Input: part model. Units: mm. Frame: model coordinates. Face numbers are marked on the shaded views. Coordinates: 2 decimals unless noted, no trailing zeros. Write each loop counter-clockwise with the first axis right and the second up, starting at its lowest first coordinate (ties: lowest second). Pieces come first, ordered by that corner, then holes. Notation, with made-up numbers: M -13,-40 L -6,-40 A6 ccw -6,-36 Z; hole C 24,-25 d2. An arc over 180 degrees is marked long. Use one line per item in the form item = value.
from build123d import *

# Parameters (mm, degrees)
SKETCH_1_R      = 46
SKETCH_1_R_2    = 20
SKETCH_1_R_3    = 3.1
EXTRUDE_1_DEPTH = 4
EXTRUDE_START   = 4
SKETCH_1_8_R    = 46
SKETCH_1_8_R_2  = 3.1
SKETCH_1_8_R_3  = 20
SKETCH_1_8_R_4  = 2.6
EXTRUDE_3_DEPTH = 6


with BuildPart() as part:
    # 草图1 → 凸台-拉伸1 (new body)
    with BuildSketch(Plane(origin=(0, 0, 0), x_dir=(1, 0, 0), z_dir=(0, 1, 0))):
        with Locations(Location((0, 0, 0), (0, 0, 270))):
            Circle(SKETCH_1_R)
        with Locations(Location((0, 0, 0), (0, 0, 270))):
            Circle(SKETCH_1_R_2, mode=Mode.SUBTRACT)
        with Locations(Location((0, 41, 0), (0, 0, 270))):
            Circle(SKETCH_1_R_3, mode=Mode.SUBTRACT)
        with Locations(Location((41, 0, 0), (0, 0, 270))):
            Circle(SKETCH_1_R_3, mode=Mode.SUBTRACT)
        with Locations(Location((0, -41, 0), (0, 0, 270))):
            Circle(SKETCH_1_R_3, mode=Mode.SUBTRACT)
        with Locations(Location((-41, 0, 0), (0, 0, 270))):
            Circle(SKETCH_1_R_3, mode=Mode.SUBTRACT)
        Polygon((-19.45, 21.16173141), (-19.45, 25.83826859), (-23.5, 28.17653718), (-27.55, 25.83826859), (-27.55, 21.16173141), (-23.5, 18.82346282), align=None, mode=Mode.SUBTRACT)
        Polygon((21.16173141, 19.45), (25.83826859, 19.45), (28.17653718, 23.5), (25.83826859, 27.55), (21.16173141, 27.55), (18.82346282, 23.5), align=None, mode=Mode.SUBTRACT)
        Polygon((19.45, -21.16173141), (19.45, -25.83826859), (23.5, -28.17653718), (27.55, -25.83826859), (27.55, -21.16173141), (23.5, -18.82346282), align=None, mode=Mode.SUBTRACT)
        Polygon((-21.16173141, -19.45), (-25.83826859, -19.45), (-28.17653718, -23.5), (-25.83826859, -27.55), (-21.16173141, -27.55), (-18.82346282, -23.5), align=None, mode=Mode.SUBTRACT)
    extrude(amount=EXTRUDE_1_DEPTH)

    # 草图1<8> → 凸台-拉伸3 (add)
    # profile 1 of 5: a face of its own
    with BuildSketch(Plane(origin=(0, 0, 0), x_dir=(1, 0, 0), z_dir=(0, 1, 0)).offset(EXTRUDE_START)):
        with Locations(Location((0, 0, 0), (0, 0, 270))):
            Circle(SKETCH_1_8_R)
        with Locations(Location((-41, 0, 0), (0, 0, 270))):
            Circle(SKETCH_1_8_R_2, mode=Mode.SUBTRACT)
        with Locations(Location((0, -41, 0), (0, 0, 270))):
            Circle(SKETCH_1_8_R_2, mode=Mode.SUBTRACT)
        with Locations(Location((41, 0, 0), (0, 0, 270))):
            Circle(SKETCH_1_8_R_2, mode=Mode.SUBTRACT)
        with Locations(Location((0, 41, 0), (0, 0, 270))):
            Circle(SKETCH_1_8_R_2, mode=Mode.SUBTRACT)
        with Locations(Location((0, 0, 0), (0, 0, 270))):
            Circle(SKETCH_1_8_R_3, mode=Mode.SUBTRACT)
        Polygon((-23.5, 18.82346282), (-19.45, 21.16173141), (-19.45, 25.83826859), (-23.5, 28.17653718), (-27.55, 25.83826859), (-27.55, 21.16173141), align=None, mode=Mode.SUBTRACT)
        Polygon((18.82346282, 23.5), (21.16173141, 19.45), (25.83826859, 19.45), (28.17653718, 23.5), (25.83826859, 27.55), (21.16173141, 27.55), align=None, mode=Mode.SUBTRACT)
        Polygon((23.5, -18.82346282), (19.45, -21.16173141), (19.45, -25.83826859), (23.5, -28.17653718), (27.55, -25.83826859), (27.55, -21.16173141), align=None, mode=Mode.SUBTRACT)
        Polygon((-18.82346282, -23.5), (-21.16173141, -19.45), (-25.83826859, -19.45), (-28.17653718, -23.5), (-25.83826859, -27.55), (-21.16173141, -27.55), align=None, mode=Mode.SUBTRACT)
    # profile 2 of 5: a face of its own
    with BuildSketch(Plane(origin=(0, 0, 0), x_dir=(1, 0, 0), z_dir=(0, 1, 0)).offset(EXTRUDE_START)):
        Polygon((-21.16173141, -27.55), (-18.82346282, -23.5), (-21.16173141, -19.45), (-25.83826859, -19.45), (-28.17653718, -23.5), (-25.83826859, -27.55), align=None)
        with Locations(Location((-23.5, -23.5, 0), (0, 0, 270))):
            Circle(SKETCH_1_8_R_4, mode=Mode.SUBTRACT)
    # profile 3 of 5: a face of its own
    with BuildSketch(Plane(origin=(0, 0, 0), x_dir=(1, 0, 0), z_dir=(0, 1, 0)).offset(EXTRUDE_START)):
        Polygon((27.55, -21.16173141), (23.5, -18.82346282), (19.45, -21.16173141), (19.45, -25.83826859), (23.5, -28.17653718), (27.55, -25.83826859), align=None)
        with Locations(Location((23.5, -23.5, 0), (0, 0, 270))):
            Circle(SKETCH_1_8_R_4, mode=Mode.SUBTRACT)
    # profile 4 of 5: a face of its own
    with BuildSketch(Plane(origin=(0, 0, 0), x_dir=(1, 0, 0), z_dir=(0, 1, 0)).offset(EXTRUDE_START)):
        Polygon((21.16173141, 27.55), (18.82346282, 23.5), (21.16173141, 19.45), (25.83826859, 19.45), (28.17653718, 23.5), (25.83826859, 27.55), align=None)
        with Locations(Location((23.5, 23.5, 0), (0, 0, 270))):
            Circle(SKETCH_1_8_R_4, mode=Mode.SUBTRACT)
    # profile 5 of 5: a face of its own
    with BuildSketch(Plane(origin=(0, 0, 0), x_dir=(1, 0, 0), z_dir=(0, 1, 0)).offset(EXTRUDE_START)):
        Polygon((-27.55, 21.16173141), (-23.5, 18.82346282), (-19.45, 21.16173141), (-19.45, 25.83826859), (-23.5, 28.17653718), (-27.55, 25.83826859), align=None)
        with Locations(Location((-23.5, 23.5, 0), (0, 0, 270))):
            Circle(SKETCH_1_8_R_4, mode=Mode.SUBTRACT)
    extrude(amount=EXTRUDE_3_DEPTH)


solid = part.part
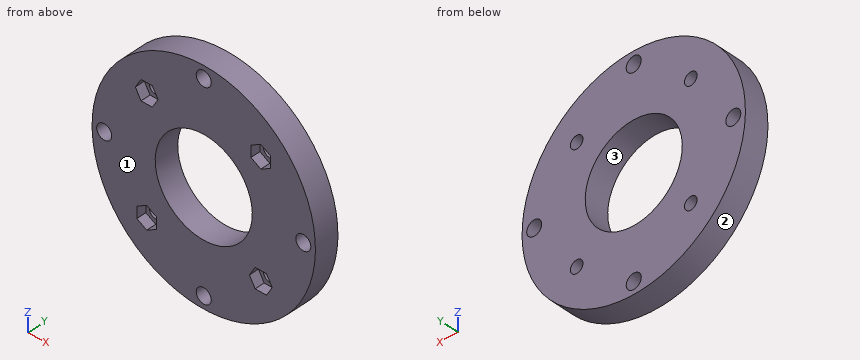
(1) Section query C-C on z = -41. Return the cut outline in (x, y), plus the area to 3 significant figures.
Computed:
outline = M -20.86,0 L -3.1,0 L -3.1,10 L -20.86,10 Z; M 3.1,0 L 20.86,0 L 20.86,10 L 3.1,10 Z
area = 355 mm^2
(2) Section query B-B on x = 0. Return the cut outline in (y, z).
Computed:
outline = M 0,-46 L 10,-46 L 10,-44.1 L 0,-44.1 Z; M 0,-37.9 L 10,-37.9 L 10,-20 L 0,-20 Z; M 0,20 L 10,20 L 10,37.9 L 0,37.9 Z; M 0,44.1 L 10,44.1 L 10,46 L 0,46 Z
(3) Section query A-A on y = 6.5. State how many separate pieces and enclosed holes the cut face has, plus the area to 3 significant figures.
Computed:
separate_pieces = 1
enclosed_holes = 9
area = 5,190 mm^2
(4) First-contact query: pin 1 Ø1.2 at (y, z) = (3, -23) entering from -X; pin 2 Ø4.5 at (x, y) = (22.5, 3) entering from -Z; pin 3 Ø2 at (x, y) = (-8.5, 8) entering from +Z; pin 4 Ø24 at (x, z) = (0, 0) entering from +Y. Flat tips, straight axial feed; report the tip coordinate or a pass-through.
Computed:
pin_1 = -40.18
pin_2 = -41.3
pin_3 = 45.38
pin_4 = through
(5) Pull-direction query (Z, two-part tool) for the marked faces 1, 2 and 3; classes: pulls with the +Z half, pulls with the -Z half, needs draft (parallel to the pull), parting line crosses it, or undercut.
Computed:
face_1 = needs draft
face_2 = parting line crosses it
face_3 = undercut
(6) Section query D-D on x = -16. Return the cut outline in (y, z).
Computed:
outline = M 0,-43.13 L 10,-43.13 L 10,-12 L 0,-12 Z; M 0,12 L 10,12 L 10,43.13 L 0,43.13 Z
(7) Line query: probe 1 along X at (y, z) = (5.85, -23.5); probe 2 along Z at (x, y) = (26.5, 3.75); probe 3 along X at (y, z) = (7.75, -24). Output: solid intervals per line, ascending.
Computed:
probe_1 = -39.54 to -26.1, -20.9 to 20.9, 26.1 to 39.54
probe_2 = -37.6 to -26.4, -20.6 to 20.56, 26.44 to 37.6
probe_3 = -39.24 to -26.05, -20.95 to 20.95, 26.05 to 39.24
